```python
from build123d import *

# Parameters (mm, degrees)
CUT_EXTRUDE_START   = -10
CUT_EXTRUDE_1_DEPTH = 10
CHAMFER_1_SIZE      = 2


with BuildPart() as part:
    # Эскиз2 → Повернуть1 (revolve)
    with BuildSketch(Plane.XY):
        Polygon((0, 0), (148, 0), (148, -12.5), (134, -12.5), (134, -15), (120, -15), (120, -28.8), (70, -28.8), (70, -18), (62, -18), (62, -15), (26, -15), (26, -12.5), (0, -12.5), align=None)
    revolve(axis=Axis((0, 0, 0), (1, 0, 0)))

    # Эскиз3 → Вырез-Повернуть1 (revolve, cut)
    with BuildSketch(Plane.XY):
        Polygon((0, 0), (10.054700538, 0), (8.9, 2), (3.9, 2), (0, 4.25), align=None)
    cut_revolve_1 = revolve(axis=Axis((0, 0, 0), (1, 0, 0)), mode=Mode.SUBTRACT)

    # Зеркальное отражение1: Вырез-Повернуть1 across plane
    add(cut_revolve_1.mirror(Plane(origin=(74, 0, 0), x_dir=(0, 0, 1), z_dir=(1, 0, 0))), mode=Mode.SUBTRACT)

    # Эскиз4 → Вырез-Вытянуть1 (cut)
    with BuildSketch(Plane.XY.offset(CUT_EXTRUDE_START)):
        with BuildLine():
            Line((37, 4), (51, 4))
            ThreePointArc((51, 4), (55, 0), (51, -4))
            Line((51, -4), (37, -4))
            ThreePointArc((37, -4), (33, 0), (37, 4))
        make_face()
    extrude(amount=-CUT_EXTRUDE_1_DEPTH, mode=Mode.SUBTRACT)

    # Фаска1
    chamfer_1_edges = [part.edges().sort_by_distance(p)[0] for p in [
        (0, 12.5, 0),
        (70, 28.8, 0),
        (120, 28.8, 0),
        (148, 12.5, 0),
    ]]
    chamfer(chamfer_1_edges, length=CHAMFER_1_SIZE)


solid = part.part
```
CAD build for the part. Positions are in the model's coordinates, mm. A direction names the side the tool comes from. Give positions to 0.01 mm unless a question says otherwise; leave off trailing zeros. Loops run counter-clockwise (first coordinate to the right, second up) from the corner with the lowest first, then second, coordinate; pieces in that order, holes last. Notation, with made-up numbers: (7.5, 34) -> (41.5, 34) arc R19 ccw to (41.5, 61) -> close; hole circle Ø8 at (-14, 79). An arc over 180 degrees is marked (long way). Use a Markdown table: item, result.
1. Which spindle directions (+Z, -Z, +X, -X, +Y, -Y) get a long thin tool onto all of the face, cutting with end or side? Do faces 1 (the cylindrical face through (55, 0, -12)), 2 (the flat face through (134, -3.4, -12.3)), 3 (the cylindrical face through (94.68, -27.47, -8.65)), 4 (the cylindrical face through (43.748, 3.252, 14.643)). Say none if no direction does.
Check result:
| item | result |
|---|---|
| face 1 | -Z |
| face 2 | +X |
| face 3 | +X, -X |
| face 4 | -X |
2. Wall check: L1, parallel to Z at x = 7.3, y = 0; L2, parallel to X at y = -3, z = 3; L3, parallel to X at y = -13, z = 17. Give the ranges that are in metal, low to high. Write a range as [from, to].
Check result:
| item | result |
|---|---|
| L1 | z = [-12.5, -2], [2, 12.5] |
| L2 | x = [0.01, 147.99] |
| L3 | x = [70, 120] |
3. Flat gauge pins, fed straight in: pin 1 (6 mm diameter, centred on x = 65, z = 6, fed in from +Y); pin 2 (3 mm diameter, centred on x = 102, z = 22, fed in from +Y); pin 3 (12 mm diameter, centred on y = 8.5, z = 21, fed in from -X); pin 4 (1.5 mm diameter, centred on x = 23.5, y = 15.5, fed in from +Z). Where does each tip first touch, or does it go through?
Check result:
| item | result |
|---|---|
| pin 1 | stops at y = 17.75 |
| pin 2 | stops at y = 20.23 |
| pin 3 | stops at x = 62 |
| pin 4 | passes through |
4. Slice it at A-A (x = 41). List the corners of the cut face in (y, z).
Check result:
| item | result |
|---|---|
| outline | (-4, -14.46) -> (-4, -10) -> (4, -10) -> (4, -14.46) arc R15 ccw (long way) to start |
5. Mould opens along X. For faces 5 (the conical face through (138.146, -0.075, -0.339)), 6 (the flat face through (44, 4, -12)), 7 (the conical face through (9.854, -0.075, -0.339)) say: pulls with the +X half, pulls with the -X half, needs draft (parallel to the pull), parting line crosses it, or undercut.
Check result:
| item | result |
|---|---|
| face 5 | pulls with the +X half |
| face 6 | undercut |
| face 7 | pulls with the -X half |
6. Slice it at B-B (x = 112). List the corners of the cut face in (y, z).
Check result:
| item | result |
|---|---|
| outline | circle Ø57.6 at (0, 0) |
7. Slice it at C-C (x = 56.5). List the corners of the cut face in (y, z).
Check result:
| item | result |
|---|---|
| outline | circle Ø30 at (0, 0) |
